from build123d import *

# Parameters (mm, degrees)
SKETCH1_R           = 3.175
BOSS_EXTRUDE1_DEPTH = 6.35
FILLET1_R           = 6.35
FILLET2_R           = 12.7
CUT_EXTRUDE1_DEPTH  = 7.35


with BuildPart() as part:
    # Sketch1 → Boss-Extrude1 (new body)
    with BuildSketch(Plane.XY):
        Polygon((0, 19.05), (0, 0), (85.725, 0), (85.725, 114.3), (66.675, 114.3), (66.675, 19.05), align=None)
        with Locations((69.85, 9.525)):
            Circle(SKETCH1_R, mode=Mode.SUBTRACT)
        with Locations((6.35, 9.525)):
            Circle(SKETCH1_R, mode=Mode.SUBTRACT)
    extrude(amount=BOSS_EXTRUDE1_DEPTH)

    # Fillet1
    fillet1_edges = [part.edges().sort_by_distance(p)[0] for p in [
        (66.675, 114.3, 3.175),
        (85.725, 114.3, 3.175),
        (85.725, 0, 3.175),
        (0, 0, 3.175),
        (0, 19.05, 3.175),
    ]]
    fillet(fillet1_edges, radius=FILLET1_R)

    # Fillet2
    fillet2_edges = [part.edges().sort_by_distance(p)[0] for p in [
        (66.675, 19.05, 3.175),
    ]]
    fillet(fillet2_edges, radius=FILLET2_R)

    # Sketch2 → Cut-Extrude1 (cut, through all)
    with BuildSketch(Plane.XY.offset(6.35)):
        with BuildLine():
            Line((53.975, 19.05), (59.055, 18.25625))
            ThreePointArc((59.055, 18.25625), (57.942186014, 18.652541864), (57.051260526, 19.42820544))
            ThreePointArc((57.051260526, 19.42820544), (55.524711116, 19.144905972), (53.975, 19.05))
        make_face()
        with BuildLine():
            ThreePointArc((57.051260526, 19.42820544), (57.942186014, 18.652541864), (59.055, 18.25625))
            ThreePointArc((59.055, 18.25625), (61.018534307, 18.580759781), (62.403160549, 20.010299477))
            ThreePointArc((62.403160549, 20.010299477), (62.639885623, 20.683811475), (62.720146595, 21.393188207))
            ThreePointArc((62.720146595, 21.393188207), (62.67970364, 21.89833881), (62.559405095, 22.390620257))
            ThreePointArc((62.559405095, 22.390620257), (59.990542874, 20.565043856), (57.051260526, 19.42820544))
        make_face()
        with BuildLine():
            ThreePointArc((62.720146595, 21.393188207), (62.639885623, 20.683811475), (62.403160549, 20.010299477))
            Line((62.403160549, 20.010299477), (65.407055815, 26.21844508))
            ThreePointArc((65.407055815, 26.21844508), (64.164589666, 24.169613306), (62.559405095, 22.390620257))
            ThreePointArc((62.559405095, 22.390620257), (62.67970364, 21.89833881), (62.720146595, 21.393188207))
        make_face()
    extrude(amount=-CUT_EXTRUDE1_DEPTH, mode=Mode.SUBTRACT)


solid = part.part
Could you check a few things on this model? Use its own coordinates, in mm. A direction names the side the tool comes from. Coordinates: 2 decimals unless noted, no trailing zeros. Write each loop counter-clockwise with the first axis right and the second up, starting at its lowest first coordinate (ties: lowest second). Pieces come first, ordered by that corner, then holes. Notation, with made-up numbers: (78.5, 53) - (122.5, 53) arc R8 ccw to (122.5, 61) - close; hole circle Ø6 at (-33.5, -7.5). An arc over 180 degrees is marked (long way). Put each result on its own line as item: value. Start each with the question number.
Q1. I'm going to push flat-ended pins straight in: P1, Ø1, axis at y = 29.5, z = 4.5, coming from the -X side; P2, Ø1.9, axis at x = 39.5, z = 2.5, coming from the +Y side; P3, Ø3, axis at y = 70, z = 4.5, coming from the -X side (3 decimals). Where does each tip first touch, or does it pass through?
Q2. I want a section at C-C on y = 37.5. Write out the boundary of the cut face in (x, z) (3 decimals).
Q3. Which directions (+Z, -Z, +X, -X, +Y, -Y) give clear straight access to the entire face, cutting with the end or side of a thin tool? Please do faces 1 (the flat face through (30, 19.05, 3)), 2 (the cylindrical face through (84, 2, 3)).
Q4. I want a section at B-B on x = 69.85. Write out the boundary of the cut face in (y, z), plus the area to 3 significant figures.
Q5. I want a section at A-A on z = 1. Write out the boundary of the cut face in (x, y) (3 decimals).
Q6. I want a section at D-D on x = 22. Write out the boundary of the cut face in (y, z), plus the area to 3 significant figures.
Q7. Thinking about a two-plate mould opening in X: for faces 3 (the flat face through (66.675, 70, 3)), 4 (the flat face through (56.48, 18.66, 3.22)), 5 (the flat face through (42, 0, 3)), 6 (the cylindrical face through (60.993, 18.568, 3.219)), which applies, pulls with the +X half, pulls with the -X half, needs draft (parallel to the pull), parting line crosses it, or undercut?
Q8. Please list where these lines run through material, in increasing order: L1, parallel to Y at x = 6.35, z = 2.25; L2, parallel to X at y = 10, z = 5 (3 decimals); L3, parallel to X at y = 106.5, z = 3.25 (3 decimals).
Checks:
1. P1: x = 66.37
1. P2: y = 19.05
1. P3: x = 66.675
2. outline: (66.675, 0) - (85.725, 0) - (85.725, 6.35) - (66.675, 6.35) - close
3. face 1: +Z, -Z, -X, +Y
3. face 2: +Z, -Z, +X, -Y
4. outline: (0, 0) - (6.35, 0) - (6.35, 6.35) - (0, 6.35) - close; (12.7, 0) - (113.45, 0) - (113.45, 6.35) - (12.7, 6.35) - close
4. area: 680 mm²
5. outline: (0, 6.35) arc R6.35 ccw to (6.35, 0) - (79.375, 0) arc R6.35 ccw to (85.725, 6.35) - (85.725, 107.95) arc R6.35 ccw to (79.375, 114.3) - (73.025, 114.3) arc R6.35 ccw to (66.675, 107.95) - (66.675, 31.75) arc R12.7 cw to (65.407, 26.218) - (62.403, 20.01) arc R3.175 cw to (59.055, 18.256) - (53.975, 19.05) - (6.35, 19.05) arc R6.35 ccw to (0, 12.7) - close; hole circle Ø6.35 at (6.35, 9.525); hole circle Ø6.35 at (69.85, 9.525)
6. outline: (0, 0) - (19.05, 0) - (19.05, 6.35) - (0, 6.35) - close
6. area: 121 mm²
7. face 3: pulls with the -X half
7. face 4: undercut
7. face 5: needs draft
7. face 6: undercut
8. L1: 0 to 6.35, 12.7 to 19.05
8. L2: 0 to 3.211, 9.489 to 66.711, 72.989 to 85.725
8. L3: 66.675 to 85.725
